```python
from build123d import *

# Parameters (mm, degrees)
BOSS_EXTRUDE1_DEPTH = 30
SKETCH2_W           = 20
SKETCH2_H           = 8
BOSS_EXTRUDE2_DEPTH = 30
BOSS_EXTRUDE3_DEPTH = 30
SKETCH5_R           = 2.778125
CUT_EXTRUDE2_DEPTH  = 112.476514483
FILLET6_R           = 2
FILLET8_R           = 3
BOSS_EXTRUDE4_START = -30
SKETCH6_W           = 100
SKETCH6_H           = 10
BOSS_EXTRUDE4_DEPTH = 30
FILLET9_R           = 5
FILLET10_R          = 5
SKETCH7_W           = 270
SKETCH7_H           = 10
BOSS_EXTRUDE5_DEPTH = 30
SKETCH8_R           = 2
CUT_EXTRUDE3_DEPTH  = 30
FILLET11_R          = 5
SKETCH9_R           = 2
CUT_EXTRUDE4_DEPTH  = 13.175


with BuildPart() as part:
    # Sketch1 → Boss-Extrude1 (new body)
    with BuildSketch(Plane.XY):
        with BuildLine():
            ThreePointArc((66.675, 0), (0, 66.675), (-66.675, 0))
            Line((-66.675, 0), (-57.15, 0))
            ThreePointArc((-57.15, 0), (0, 57.15), (57.15, 0))
            Line((57.15, 0), (66.675, 0))
        make_face()
    extrude(amount=BOSS_EXTRUDE1_DEPTH)

    # Sketch2 → Boss-Extrude2 (add)
    with BuildSketch(Plane.XY.offset(30)):
        with Locations((-71.9125, 4)):
            Rectangle(SKETCH2_W, SKETCH2_H)
        with Locations((71.9125, 4)):
            Rectangle(SKETCH2_W, SKETCH2_H)
    extrude(amount=-BOSS_EXTRUDE2_DEPTH)

    # Sketch4 → Boss-Extrude3 (add)
    with BuildSketch(Plane.XY.offset(30)):
        Polygon((-89.9125, 0), (-81.9125, 0), (-81.9125, 35), (-40.473552557, 47.215668719), (-30.223695263, 59.431337438), (-89.9125, 35), align=None)
        Polygon((30.223695263, 59.431337438), (40.473552557, 47.215668719), (81.9125, 35), (81.9125, 0), (89.9125, 0), (89.9125, 35), align=None)
    extrude(amount=-BOSS_EXTRUDE3_DEPTH)

    # Sketch5 → Cut-Extrude2 (cut, through all)
    with BuildSketch(Plane(origin=(0, 8, 0), x_dir=(1, 0, 0), z_dir=(0, 1, 0))):
        with Locations(Location((-74.052910047, -15, 0), (0, 0, 180))):
            Circle(SKETCH5_R)
        with Locations((74.052910047, -15)):
            Circle(SKETCH5_R)
    extrude(amount=-CUT_EXTRUDE2_DEPTH, mode=Mode.SUBTRACT)

    # Fillet6
    fillet6_edges = [part.edges().sort_by_distance(p)[0] for p in [
        (-81.9125, 8, 15),
        (-66.193320093, 8, 15),
        (66.193320093, 8, 15),
        (81.9125, 8, 15),
    ]]
    fillet(fillet6_edges, radius=FILLET6_R)

    # Fillet7
    # a fillet whose section is not a circle: 20, 15 mm, written as the material it adds along each edge
    with BuildSketch(Plane(origin=(81.9125, 35, 30), x_dir=(-0.9591914836749359, 0.28275731227587253, 0), z_dir=(0, 0, -1))) as fillet7_piece_1:
        with BuildLine():
            Bezier((16.42908698, 0), (0, 0), (-2.754742693, -9.344853754), weights=[1, 0.800861197, 1])
            Line((-2.754742693, -9.344853754), (0, 0))
            Line((0, 0), (16.42908698, 0))
        make_face()
    extrude(amount=30)
    with BuildSketch(Plane(origin=(-81.9125, 35, 30), x_dir=(0, -1, 0), z_dir=(0, 0, -1))) as fillet7_piece_2:
        with BuildLine():
            Bezier((9.742427777, 0), (0, 0), (-4.645444478, -15.758640316), weights=[1, 0.800861197, 1])
            Line((-4.645444478, -15.758640316), (0, 0))
            Line((0, 0), (9.742427777, 0))
        make_face()
    extrude(amount=30)
    # a fillet whose section is not a circle: 20, 15 mm, written as the material it takes off along each edge
    with BuildSketch(Plane(origin=(89.9125, 35, 68.677099201), x_dir=(0, -1, 0), z_dir=(0, 0, -1))) as fillet7_2_piece_1:
        with BuildLine():
            Bezier((8.021650729, 0), (0, 0), (-5.860478322, 14.317879531), weights=[1, 0.830303568, 1])
            Line((-5.860478322, 14.317879531), (0, 0))
            Line((0, 0), (8.021650729, 0))
        make_face()
    extrude(amount=107.354198402, mode=Mode.SUBTRACT)
    with BuildSketch(Plane(origin=(-89.9125, 35, 68.677099201), x_dir=(0.9254752700268907, 0.37880803128847984, 0), z_dir=(0, 0, -1))) as fillet7_2_piece_2:
        with BuildLine():
            Bezier((15.47083968, 0), (0, 0), (-3.03866572, 7.423839374), weights=[1, 0.830303568, 1])
            Line((-3.03866572, 7.423839374), (0, 0))
            Line((0, 0), (15.47083968, 0))
        make_face()
    extrude(amount=107.354198402, mode=Mode.SUBTRACT)

    # Fillet8
    fillet8_edges = [part.edges().sort_by_distance(p)[0] for p in [
        (-49.639626869, 44.513627906, 15),
        (49.639626869, 44.513627906, 15),
    ]]
    fillet(fillet8_edges, radius=FILLET8_R)

    # Sketch6 → Boss-Extrude4 (add)
    with BuildSketch(Plane.XY.offset(30).offset(BOSS_EXTRUDE4_START)):
        with Locations((0, 81.675)):
            Rectangle(SKETCH6_W, SKETCH6_H)
        Polygon((-43.476507509, 76.675), (-50, 76.675), (-60.5630878, 47.013063358), (-50.022382459, 51.327499376), align=None)
        with BuildLine():
            Line((12.5, 76.675), (-12.5, 76.675))
            Line((-12.5, 76.675), (-12.5, 65.492790634))
            ThreePointArc((-12.5, 65.492790634), (0, 66.675), (12.5, 65.492790634))
            Line((12.5, 65.492790634), (12.5, 76.675))
        make_face()
        Polygon((60.5630878, 47.013063358), (50, 76.675), (43.476507509, 76.675), (50.022382459, 51.327499376), align=None)
    extrude(amount=BOSS_EXTRUDE4_DEPTH)

    # Fillet9
    fillet9_edges = [part.edges().sort_by_distance(p)[0] for p in [
        (43.476507509, 76.675, 15),
        (12.5, 76.675, 15),
        (12.5, 65.492790634, 15),
        (-12.5, 65.492790634, 15),
        (-12.5, 76.675, 15),
        (-43.476507509, 76.675, 15),
    ]]
    fillet(fillet9_edges, radius=FILLET9_R)

    # Fillet10
    fillet10_edges = [part.edges().sort_by_distance(p)[0] for p in [
        (-50.022382459, 51.327499376, 15),
        (50.022382459, 51.327499376, 15),
    ]]
    fillet(fillet10_edges, radius=FILLET10_R)

    # Sketch7 → Boss-Extrude5 (add)
    with BuildSketch(Plane.XY.offset(30)):
        with Locations((0, 81.675)):
            Rectangle(SKETCH7_W, SKETCH7_H)
    extrude(amount=-BOSS_EXTRUDE5_DEPTH)

    # Sketch8 → Cut-Extrude3 (cut)
    with BuildSketch(Plane(origin=(0, 86.675, 0), x_dir=(1, 0, 0), z_dir=(0, 1, 0))):
        with Locations(Location((130, -15, 0), (0, 0, 180))):
            Circle(SKETCH8_R)
        with Locations(Location((120, -15, 0), (0, 0, 180))):
            Circle(SKETCH8_R)
        with Locations(Location((-120, -15, 0), (0, 0, 90))):
            Circle(SKETCH8_R)
        with Locations(Location((-130, -15, 0), (0, 0, 90))):
            Circle(SKETCH8_R)
    extrude(amount=-CUT_EXTRUDE3_DEPTH, mode=Mode.SUBTRACT)

    # Fillet11
    fillet11_edges = [part.edges().sort_by_distance(p)[0] for p in [
        (135, 81.675, 30),
        (-135, 81.675, 0),
        (135, 81.675, 0),
        (-135, 81.675, 30),
    ]]
    fillet(fillet11_edges, radius=FILLET11_R)

    # Sketch9 → Cut-Extrude4 (cut)
    with BuildSketch(Plane(origin=(0, 86.675, 0), x_dir=(1, 0, 0), z_dir=(0, 1, 0))):
        with Locations(Location((27, -15, 0), (0, 0, 180))):
            Circle(SKETCH9_R)
        with Locations(Location((-27, -15, 0), (0, 0, 180))):
            Circle(SKETCH9_R)
    extrude(amount=-CUT_EXTRUDE4_DEPTH, mode=Mode.SUBTRACT)


solid = part.part
```
Source: CAD feature listing. Evaluate the final solid. Frame: model axes, mm. A direction names the side the tool comes from. Coordinates: 2 decimals unless noted, no trailing zeros. Write each loop counter-clockwise with the first axis right and the second up, starting at its lowest first coordinate (ties: lowest second). Pieces come first, ordered by that corner, then holes. Notation, with made-up numbers: (66.5, 33) -> (110.5, 33) arc R25 cw to (110.5, 53) -> close; hole circle Ø4 at (43, 87). An arc over 180 degrees is marked (long way). Return JSON: item names as keys, results as strings. Group by question number.
1) Section query D-D, the plane x = -100. Return loops of the section in (y, z) (3 decimals).
2) Section query B-B, the plane x = -36. Return loops of the section in (y, z) (3 decimals), plus the area to 3 significant figures.
3) Section query A-A, the plane y = 52. Return loops of the section in (x, z), plus the area to 3 significant figures.
4) Contact query for flat-ended pins moving along their axis: P1, Ø5, axis at y = 27, z = 3.5, coming from the -X side; P2, Ø8, axis at y = 22, z = 19.5, coming from the +X side; P3, Ø15, axis at x = 112, z = 20.5, coming from the -Y side (3 decimals). Output: stop coordinate, or through.
5) Ray query, line 1 along X through (y, z) = (74, 8); line 2 along Z through (x, y) = (120, 82); line 3 along X through (y, z) = (16.5, 10.5). Return the intervals inside material, ascending.
6) Section query C-C, the plane y = 19. Return loops of the section in (x, z).
7) Mould query, pull axis Z, two halves, no side actions, for faces 1 (the face through (-71.277, 4.056, 15.122)), 2 (the face through (-1, 63, 0)), 3 (the face through (-134, 82, 28)), 4 (the face through (71, 8, 15)). Classes: +Z half, -Z half, draft (parallel to the pull), parting line (faces both ways), or undercut.
8) Set-up query: faces 5 (the face through (-55.21, 62.05, 14.79)), 6 (the face through (-135, 82, 15)), 7 (the face through (-23.3, 62.47, 14.79)), 8 (the face through (68.184, 43.894, 15.21)). Return all of +Z, -Z, +X, -X, +Y, -Y with unobstructed straight access to the full face (end or side cutting, diameter ignored); none if empty.
From the geometry:
{
 "1": {"outline": "(76.675, 0) -> (86.675, 0) -> (86.675, 30) -> (76.675, 30) -> close"},
 "2": {"outline": "(44.386, 0) -> (57.067, 0) -> (57.067, 30) -> (44.386, 30) -> close; (76.675, 0) -> (86.675, 0) -> (86.675, 30) -> (76.675, 30) -> close", "area": "680 mm²"},
 "3": {"outline": "(-58.79, 0) -> (-23.71, 0) -> (-23.71, 30) -> (-58.79, 30) -> close; (23.71, 0) -> (58.79, 0) -> (58.79, 30) -> (23.71, 30) -> close", "area": "2,100 mm²"},
 "4": {"P1": "x = -89.91", "P2": "x = 89.91", "P3": "y = 76.675"},
 "5": {"line 1": "-50.95 to -44.03, -13.07 to 13.07, 44.03 to 50.95", "line 2": "0 to 13, 17 to 30", "line 3": "-89.91 to -81.91, -64.6 to -54.72, 54.72 to 64.6, 81.91 to 89.91"},
 "6": {"outline": "(-89.91, 0) -> (-81.91, 0) -> (-81.91, 30) -> (-89.91, 30) -> close; (-63.91, 0) -> (-53.9, 0) -> (-53.9, 30) -> (-63.91, 30) -> close; (53.9, 0) -> (63.91, 0) -> (63.91, 30) -> (53.9, 30) -> close; (81.91, 0) -> (89.91, 0) -> (89.91, 30) -> (81.91, 30) -> close"},
 "7": {"face 1": "undercut", "face 2": "-Z half", "face 3": "+Z half", "face 4": "draft"},
 "8": {"face 5": "+Z, -Z, -X", "face 6": "+Z, -Z, -X, +Y, -Y", "face 7": "+Z, -Z", "face 8": "+Z, -Z, +X"}
}
